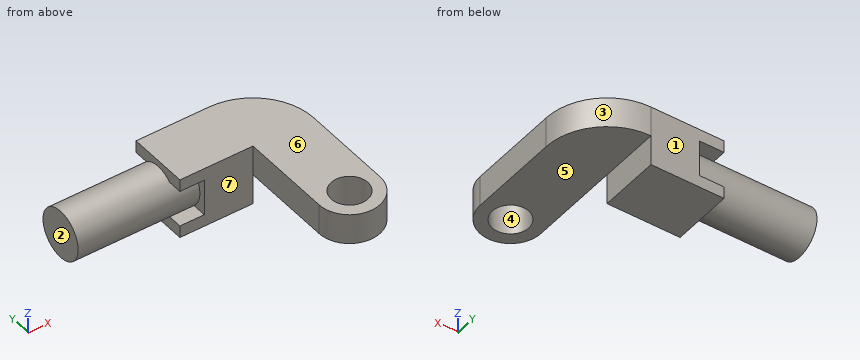
```python
from build123d import *

# Parameters (mm, degrees)
SKETCH2_R           = 12.7
BOSS_EXTRUDE1_DEPTH = 63.5
SKETCH3_W           = 31.75
SKETCH3_H           = 31.75
BOSS_EXTRUDE2_DEPTH = 25.4
SKETCH6_W           = 12.7
SKETCH6_H           = 31.75
BOSS_EXTRUDE3_DEPTH = 6.35
SKETCH7_R           = 9.525
BOSS_EXTRUDE4_DEPTH = 15.875


with BuildPart() as part:
    # Sketch2 → Boss-Extrude1 (new body)
    with BuildSketch(Plane(origin=(0, 0, 0), x_dir=(0, 0, -1), z_dir=(1, 0, 0))):
        Circle(SKETCH2_R)
    extrude(amount=BOSS_EXTRUDE1_DEPTH)

    # Sketch3 → Boss-Extrude2 (add)
    with BuildSketch(Plane(origin=(63.5, 0, 0), x_dir=(0, 0, -1), z_dir=(1, 0, 0))):
        Rectangle(SKETCH3_W, SKETCH3_H)
    extrude(amount=BOSS_EXTRUDE2_DEPTH)

    # Sketch6 → Boss-Extrude3 (add)
    with BuildSketch(Plane(origin=(0, 0, -15.875), x_dir=(-1, 0, 0), z_dir=(0, 0, -1))):
        with Locations((-57.15, 0)):
            Rectangle(SKETCH6_W, SKETCH6_H)
    boss_extrude3 = extrude(amount=-BOSS_EXTRUDE3_DEPTH)

    # Mirror1: Boss-Extrude3 across plane
    add(boss_extrude3.mirror(Plane.XY))

    # Sketch7 → Boss-Extrude4 (add)
    with BuildSketch(Plane.XY.offset(15.875)):
        with BuildLine():
            Line((88.9, 15.875), (88.9, -63.627))
            ThreePointArc((88.9, -63.627), (104.775, -79.502), (120.65, -63.627))
            Line((120.65, -63.627), (120.65, -15.875))
            ThreePointArc((120.65, -15.875), (111.350640303, 6.575640303), (88.9, 15.875))
        make_face()
        with Locations((104.775, -63.627)):
            Circle(SKETCH7_R, mode=Mode.SUBTRACT)
    extrude(amount=-BOSS_EXTRUDE4_DEPTH)


solid = part.part
```
For this review, take the finished solid that the model builds, in its own axes (mm). Face numbers are marked on the shaded views. A direction names the side the tool comes from. Coordinates: 2 decimals unless noted, no trailing zeros. Write each loop counter-clockwise with the first axis right and the second up, starting at its lowest first coordinate (ties: lowest second). Pieces come first, ordered by that corner, then holes. Notation, with made-up numbers: (47.5, -1) - (97.5, -1) arc R15 ccw to (97.5, 26) - close; hole circle Ø4 at (-39.75, 47). An arc over 180 degrees is marked (long way). Answer in a Markdown table with one row per item. Add a question column.
Q1. Draft analysis for pull direction X (two halves, no side actions). For the marked faces 1, 2, 3 and 4, state which applies: +X half, -X half, draft (parallel to the pull), parting line (faces both ways), or undercut.
Q2. We need section B-B, the plane z = 5. State the section outline as (x, y) points (3 decimals), and give its area (3 significant figures).
Q3. For P1, Ø2, axis at y = 0.5, z = 6, coming from the -X side; P2, Ø17, axis at x = 104.775, y = -63.627, coming from the +Z side; P3, Ø5, axis at x = 83, z = 3.5, coming from the -Y side (3 decimals); P4, Ø5, axis at y = -1, z = -7.5, coming from the +X side, all flat-tipped, find the tip position at first contact; note any pin that passes through.
Q4. We need section C-C, the plane x = 97. State the section outline as (y, z) points (3 decimals).
Q5. For probe 1 along X at (y, z) = (-63.5, 6); probe 2 along Y at (x, z) = (68.5, 9) (3 decimals); probe 3 along X at (y, z) = (-16.5, 13), list the stretches that pass through material, from the lowest coordinate up.
Q6. We need section A-A, the plane x = 61. State the section outline as (y, z) points (3 decimals), and give its area (3 significant figures).
Q7. Tool access review of the marked faces 5, 6 and 7: name each direction out of +Z, -Z, +X, -X, +Y, -Y from which nothing blocks a thin tool from reaching the whole face with its end or side.
Q8. We need section D-D, the plane y = 0. State the section outline as (x, z) points (3 decimals).
Answer list:
| question | item | result |
|---|---|---|
| 1 | face 1 | draft |
| 1 | face 2 | -X half |
| 1 | face 3 | +X half |
| 1 | face 4 | undercut |
| 2 | outline | (0, -11.674) - (63.5, -11.674) - (63.5, -15.875) - (88.9, -15.875) - (88.9, -63.627) arc R15.875 ccw to (120.65, -63.627) - (120.65, -15.875) arc R31.75 ccw to (88.9, 15.875) - (63.5, 15.875) - (63.5, 11.674) - (0, 11.674) - close; hole circle Ø19.05 at (104.775, -63.627) |
| 2 | area | 4,710 mm2 |
| 3 | P1 | stops at x = 0 |
| 3 | P2 | passes through |
| 3 | P3 | stops at y = -15.875 |
| 3 | P4 | stops at x = 88.9 |
| 4 | outline | (-77.468, 0) - (-69.129, 0) - (-69.129, 15.875) - (-77.468, 15.875) - close; (-58.125, 0) - (14.824, 0) - (14.824, 15.875) - (-58.125, 15.875) - close |
| 5 | probe 1 | x = 88.9 to 95.25, 114.3 to 120.65 |
| 5 | probe 2 | y = -15.875 to 15.875 |
| 5 | probe 3 | x = 88.9 to 120.65 |
| 6 | outline | (-15.875, -15.875) - (15.875, -15.875) - (15.875, -9.525) - (8.4, -9.525) arc R12.7 ccw to (8.4, 9.525) - (15.875, 9.525) - (15.875, 15.875) - (-15.875, 15.875) - (-15.875, 9.525) - (-8.4, 9.525) arc R12.7 ccw to (-8.4, -9.525) - (-15.875, -9.525) - close |
| 6 | area | 837 mm2 |
| 7 | face 5 | -Z, +X, +Y, -Y |
| 7 | face 6 | +Z, +X, -X, +Y, -Y |
| 7 | face 7 | +Z, -Z, -X, -Y |
| 8 | outline | (0, -12.7) - (50.8, -12.7) - (50.8, -15.875) - (88.9, -15.875) - (88.9, 0) - (116.396, 0) - (116.396, 15.875) - (50.8, 15.875) - (50.8, 12.7) - (0, 12.7) - close |
